Here's the drawing with two shaded views (mm, measured from the low corner). I have some questions. Coordinates: 2 decimals unless noted, no trailing zeros. Write each loop counter-clockwise with the first axis right and the second up, starting at its lowest first coordinate (ties: lowest second). Pieces come first, ordered by that corner, then holes. Notation, with made-up numbers: M 78,26.25 L 84,26.25 A30 ccw 84,64.25 Z; hole C 33.25,59.25 d3. An arc over 180 degrees is marked long. Answer as CSV lines item,"result". Start each with the question number.
Item 1: Suppose I cut it at B-B, the plane x = 25.5. Write out the boundary of the cut face in (y, z).
Item 2: Suppose I cut it at C-C, the plane y = 164.5. Write out the boundary of the cut face in (x, z), and give its area (3 significant figures).
Item 3: Suppose I cut it at A-A, the plane z = 30.5. Write out the boundary of the cut face in (x, y).
Item 4: I'm going to push flat-ended pins straight in: P1, Ø6, axis at y = 255.5, z = 62, coming from the -X side (1 decimal); P2, Ø6, axis at y = 121.5, z = 69.5, coming from the +X side; P3, Ø4, axis at x = 21.5, y = 224.5, coming from the +Z side; P4, Ø6, axis at x = 67.5, z = 13, coming from the -Y side. Where does each tip first touch, or does it pass through?
Item 5: If I drill on line 1 along X through (y, z) = (239, 47) (1 decimal); line 2 along Z through (x, y) = (23, 251) (1 decimal); line 3 along Z through (x, y) = (68, 54) (1 decimal), over which ranges is the centre line in solid material (lowest first)? Write a range as [from, to].
Item 6: We'd pull the mould along X, two halves only. Please class the marked faces 1 and 2: +X half, -X half, draft (parallel to the pull), parting line (faces both ways), or undercut.
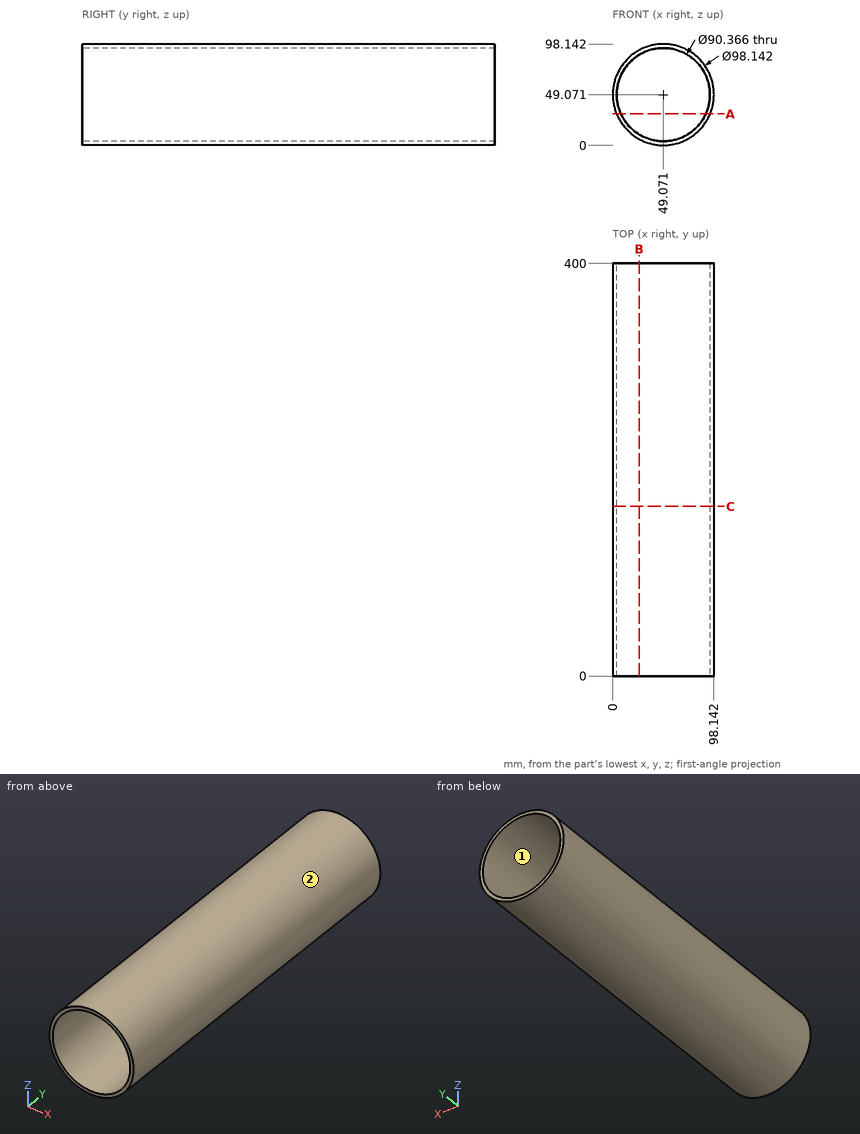
Ans:
1,outline,"M 0,6.03 L 400,6.03 L 400,10.52 L 0,10.52 Z; M 0,87.62 L 400,87.62 L 400,92.11 L 0,92.11 Z"
2,outline,"C 49.07,49.07 d98.14; hole C 49.07,49.07 d90.37"
2,area,"1,150 mm^2"
3,outline,"M 3.65,0 L 7.88,0 L 7.88,400 L 3.65,400 Z; M 90.26,0 L 94.49,0 L 94.49,400 L 90.26,400 Z"
4,P1,"stops at x = 1"
4,P2,"stops at x = 94.94"
4,P3,"stops at z = 90.95"
4,P4,"passes through"
5,line 1,"x = [0, 3.9], [94.2, 98.1]"
5,line 2,"z = [7.5, 12.2], [86, 90.6]"
5,line 3,"z = [3.8, 8], [90.1, 94.3]"
6,face 1,"undercut"
6,face 2,"parting line"
